The model under review builds one solid part; all positions refer to its coordinate system, in mm. Coordinates: 2 decimals unless noted, no trailing zeros. Order: outer loops, then holes, each group sorted by start corner. A loop starts at its lowest first (then second) coordinate and runs counter-clockwise, first axis right, second up. Notation, with made-up numbers: (28.5, -36.5) -> (60.5, -36.5) arc R19 cw to (60.5, -0.5) -> close; hole circle Ø6 at (-5.75, 63.5). An arc over 180 degrees is marked (long way). Use one line per item in the form item = value.
from build123d import *

# Parameters (mm, degrees)
BASE_FLANGE1_DEPTH  = 3
SKETCH7_W           = 25.2
SKETCH7_H           = 2.55
CUT_EXTRUDE1_DEPTH  = 10
SKETCH8_W           = 3
SKETCH8_H           = 25
BOSS_EXTRUDE1_DEPTH = 3
SKETCH9_W           = 0.35
SKETCH9_H           = 20
SKETCH9_H_2         = 23.55
CUT_EXTRUDE2_DEPTH  = 4.55
CUT_EXTRUDE3_START  = -4.55
CUT_EXTRUDE3_DEPTH  = 4.55
SKETCH11_R          = 2.5
CUT_EXTRUDE4_DEPTH  = 238.069747121


# Sheet-metal steps are written as plain solids
with BuildPart() as part:
    # Sketch1 → Base-Flange1 (new body)
    with BuildSketch(Plane(origin=(0, 0, 0), x_dir=(1, 0, 0), z_dir=(0, 1, 0))):
        with BuildLine():
            Line((-219.25, 79.3), (219.25, 79.3))
            Line((219.25, 79.3), (219.25, -79.3))
            ThreePointArc((219.25, -79.3), (218.224873734, -81.774873734), (215.75, -82.8))
            Line((215.75, -82.8), (-215.75, -82.8))
            ThreePointArc((-215.75, -82.8), (-218.224873734, -81.774873734), (-219.25, -79.3))
            Line((-219.25, -79.3), (-219.25, 79.3))
        make_face()
        with BuildLine():
            Line((-195.2, 60.25), (195.2, 60.25))
            ThreePointArc((195.2, 60.25), (198.735533906, 58.785533906), (200.2, 55.25))
            Line((200.2, 55.25), (200.2, -58.75))
            ThreePointArc((200.2, -58.75), (198.735533906, -62.285533906), (195.2, -63.75))
            Line((195.2, -63.75), (-195.2, -63.75))
            ThreePointArc((-195.2, -63.75), (-198.735533906, -62.285533906), (-200.2, -58.75))
            Line((-200.2, -58.75), (-200.2, 55.25))
            ThreePointArc((-200.2, 55.25), (-198.735533906, 58.785533906), (-195.2, 60.25))
        make_face(mode=Mode.SUBTRACT)
    extrude(amount=-BASE_FLANGE1_DEPTH)

    # Sketch7 → Cut-Extrude1 (cut)
    with BuildSketch(Plane.XZ.offset(3)):
        with Locations((186.75, -78.025)):
            Rectangle(SKETCH7_W, SKETCH7_H)
        with Locations((93.375, -78.025)):
            Rectangle(SKETCH7_W, SKETCH7_H)
        with Locations((0, -78.025)):
            Rectangle(SKETCH7_W, SKETCH7_H)
        with Locations((-93.375, -78.025)):
            Rectangle(SKETCH7_W, SKETCH7_H)
        with Locations((-186.75, -78.025)):
            Rectangle(SKETCH7_W, SKETCH7_H)
    extrude(amount=-CUT_EXTRUDE1_DEPTH, mode=Mode.SUBTRACT)

    # Sketch8 → Boss-Extrude1 (add)
    with BuildSketch(Plane.XZ.offset(3)):
        with Locations((-220.75, -46.8)):
            Rectangle(SKETCH8_W, SKETCH8_H)
        with Locations((-220.75, 1.75)):
            Rectangle(SKETCH8_W, SKETCH8_H)
        with Locations((-220.75, 50.3)):
            Rectangle(SKETCH8_W, SKETCH8_H)
    boss_extrude1 = extrude(amount=-BOSS_EXTRUDE1_DEPTH)

    # Sketch9 → Cut-Extrude2 (cut)
    with BuildSketch(Plane.XZ.offset(3)):
        with Locations((-219.075, -69.3)):
            Rectangle(SKETCH9_W, SKETCH9_H)
        with Locations((-219.075, -22.525)):
            Rectangle(SKETCH9_W, SKETCH9_H_2)
        with Locations((-219.075, 26.025)):
            Rectangle(SKETCH9_W, SKETCH9_H_2)
    cut_extrude2 = extrude(amount=-CUT_EXTRUDE2_DEPTH, mode=Mode.SUBTRACT)

    # Mirror1: Boss-Extrude1, Cut-Extrude2 across plane
    add(boss_extrude1.mirror(Plane(origin=(0, 0, 0), x_dir=(0, 0, 1), z_dir=(1, 0, 0))))
    add(cut_extrude2.mirror(Plane(origin=(0, 0, 0), x_dir=(0, 0, 1), z_dir=(1, 0, 0))), mode=Mode.SUBTRACT)

    # Sketch10 → Cut-Extrude3 (cut)
    with BuildSketch(Plane.XZ.offset(3).offset(CUT_EXTRUDE3_START)):
        with BuildLine():
            Line((219.25, 79.3), (219.25, 62.8))
            Line((219.25, 62.8), (218.9, 62.8))
            Line((218.9, 62.8), (218.9, 79.3))
            ThreePointArc((218.9, 79.3), (217.977386361, 81.527386361), (215.75, 82.45))
            Line((215.75, 82.45), (-215.75, 82.45))
            ThreePointArc((-215.75, 82.45), (-217.977386361, 81.527386361), (-218.9, 79.3))
            Line((-218.9, 79.3), (-218.9, 62.8))
            Line((-218.9, 62.8), (-219.25, 62.8))
            Line((-219.25, 62.8), (-219.25, 79.3))
            ThreePointArc((-219.25, 79.3), (-218.224873734, 81.774873734), (-215.75, 82.8))
            Line((-215.75, 82.8), (215.75, 82.8))
            ThreePointArc((215.75, 82.8), (218.224873734, 81.774873734), (219.25, 79.3))
        make_face()
    extrude(amount=CUT_EXTRUDE3_DEPTH, mode=Mode.SUBTRACT)

    # Sketch11 → Cut-Extrude4 (cut, through all)
    with BuildSketch(Plane.XZ.offset(3)):
        with Locations(Location((-119.740950076, 76.275, 0), (0, 0, 270))):
            Circle(SKETCH11_R)
        with Locations(Location((-119.740950076, -69.775, 0), (0, 0, 270))):
            Circle(SKETCH11_R)
        with Locations(Location((119.860899699, -69.775, 0), (0, 0, 270))):
            Circle(SKETCH11_R)
        with Locations(Location((119.860899699, 76.275, 0), (0, 0, 270))):
            Circle(SKETCH11_R)
    extrude(amount=-CUT_EXTRUDE4_DEPTH, mode=Mode.SUBTRACT)


solid = part.part
Item 1: We need section A-A (z = 0.5). Write out the cut boundary in (x, y).
Results found:
outline = (-222.25, -3) -> (-200.2, -3) -> (-200.2, 0) -> (-222.25, 0) -> close; (200.2, -3) -> (222.25, -3) -> (222.25, 0) -> (200.2, 0) -> close
Item 2: We need section B-B (x = 89). Write out the cut boundary in (y, z), plus the area to 3 significant figures.
Results found:
outline = (-3, -76.75) -> (0, -76.75) -> (0, -60.25) -> (-3, -60.25) -> close; (-3, 63.75) -> (0, 63.75) -> (0, 82.45) -> (-3, 82.45) -> close
area = 106 mm²
Item 3: Clearance check with flat-ended pins moving along their axes: pin 1 (1.5 mm diameter, centred on x = 220, y = -1, fed in from +Z); pin 2 (0.8 mm diameter, centred on y = -1, z = -78.5, fed in from +X); pin 3 (1.5 mm diameter, centred on x = -187.5, y = -1.5, fed in from -Z). State where each tip first meets the part, or that it passes through.
Results found:
pin_1 = 62.8
pin_2 = 218.9
pin_3 = -76.75
Item 4: To check wall thickness, follow L1, parallel to Z at x = 145, y = -0.8; L2, parallel to X at y = -0.6, z = -19; L3, parallel to X at y = -2.55, z = 52. State the ranges of each line that lie inside material, in increasing order. Write a range as from..to.
Results found:
L1 = -79.3..-60.25, 63.75..82.45
L2 = -218.9..-200.2, 200.2..218.9
L3 = -222.25..-200.2, 200.2..222.25
Item 5: We need section C-C (y = -1.75). State how many separate pieces and enclosed holes the cut face has, plus the area to 3 significant figures.
Results found:
separate_pieces = 1
enclosed_holes = 5
area = 21,300 mm²
